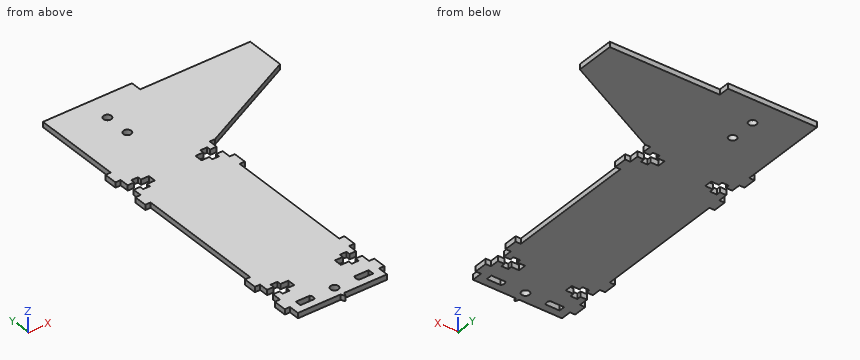
```python
from build123d import *

# Parameters (mm, degrees)
SKETCH_1_R      = 1.5
EXTRUDE_1_DEPTH = 2


with BuildPart() as part:
    # 草图1 → 凸台-拉伸1 (new body)
    with BuildSketch(Plane.XY):
        Polygon((16.993865071, 15.9), (16.993865071, 20), (-16.993865071, 20), (-16.993865071, 15.9), (-16.993865071, -14), (-18.993865071, -14), (-18.993865071, -19), (-16.993865071, -19), (-16.993865071, -22.5), (-14.493865071, -22.5), (-14.493865071, -21), (-11.893865071, -21), (-11.893865071, -22.5), (-8.893865071, -22.5), (-8.893865071, -25.5), (-11.893865071, -25.5), (-11.893865071, -27), (-14.493865071, -27), (-14.493865071, -25.5), (-16.993865071, -25.5), (-16.993865071, -29), (-18.993865071, -29), (-18.993865071, -34), (-16.993865071, -34), (-16.993865071, -84), (-18.993865071, -84), (-18.993865071, -89), (-16.993865071, -89), (-16.993865071, -92.5), (-14.493865071, -92.5), (-14.493865071, -91), (-11.893865071, -91), (-11.893865071, -92.5), (-8.893865071, -92.5), (-8.893865071, -95.5), (-11.893865071, -95.5), (-11.893865071, -97), (-14.493865071, -97), (-14.493865071, -95.5), (-16.993865071, -95.5), (-16.993865071, -99), (-18.993865071, -99), (-18.993865071, -104), (-16.993865071, -104), (-16.993865071, -108), (-0.721190694, -108), (0, -109.5), (0.721190694, -108), (16.993865071, -108), (16.993865071, -104), (18.993865071, -104), (18.993865071, -99), (16.993865071, -99), (16.993865071, -95.5), (14.493865071, -95.5), (14.493865071, -97), (11.893865071, -97), (11.893865071, -95.5), (8.893865071, -95.5), (8.893865071, -92.5), (11.893865071, -92.5), (11.893865071, -91), (14.493865071, -91), (14.493865071, -92.5), (16.993865071, -92.5), (16.993865071, -89), (18.993865071, -89), (18.993865071, -84), (16.993865071, -84), (16.993865071, -34), (18.993865071, -34), (18.993865071, -29), (16.993865071, -29), (16.993865071, -25.5), (14.493865071, -25.5), (14.493865071, -27), (11.893865071, -27), (11.893865071, -25.5), (8.893865071, -25.5), (8.893865071, -22.5), (11.893865071, -22.5), (11.893865071, -21), (14.493865071, -21), (14.493865071, -22.5), (16.993865071, -22.5), (16.993865071, -19), (18.993865071, -19), (58.993865071, 0.9), (58.993865071, 15.9), align=None)
        with Locations((0, -104)):
            Circle(SKETCH_1_R, mode=Mode.SUBTRACT)
        Circle(SKETCH_1_R, mode=Mode.SUBTRACT)
        with Locations((0, 10)):
            Circle(SKETCH_1_R, mode=Mode.SUBTRACT)
        with BuildLine():
            Line((-13.9, -102.85), (-8.6, -102.85))
            ThreePointArc((-8.6, -102.85), (-8.123654403, -104), (-8.6, -105.15))
            Line((-8.6, -105.15), (-13.9, -105.15))
            Line((-13.9, -105.15), (-13.9, -102.85))
        make_face(mode=Mode.SUBTRACT)
        with BuildLine():
            Line((13.9, -105.15), (8.6, -105.15))
            ThreePointArc((8.6, -105.15), (8.123654403, -104), (8.6, -102.85))
            Line((8.6, -102.85), (13.9, -102.85))
            Line((13.9, -102.85), (13.9, -105.15))
        make_face(mode=Mode.SUBTRACT)
    extrude(amount=EXTRUDE_1_DEPTH)


solid = part.part
```
Design review of the part built by this model. Coordinates are the model's own, in mm. Give positions to 0.01 mm unless a question says otherwise; leave off trailing zeros. Loops run counter-clockwise (first coordinate to the right, second up) from the corner with the lowest first, then second, coordinate; pieces in that order, holes last. Notation, with made-up numbers: M 38.5,1 L 84.5,1 A21 ccw 84.5,8 Z; hole C -24,-23.5 d5. An arc over 180 degrees is marked long. Return JSON: item names as keys, results as strings. Group by question number.
Item 1: We need section A-A (y = 10). Give the boundary of the cut face in (x, z), and give its area (3 significant figures).
Item 2: We need section C-C (z = 1.6). Give the number of separate pieces and of enclosed holes in the cut face, and give its area (3 significant figures).
Item 3: For probe 1 along Y at (x, z) = (18.5, 1.9); probe 2 along Y at (x, z) = (9, 1.4); probe 3 along X at (y, z) = (-96, 0.35), list the stretches that pass through material, from the lowest coordinate up.
Item 4: Insertion check: pin 1 Ø0.6 at (x, z) = (-16, 1) entering from -Y; pin 2 Ø0.6 at (y, z) = (-32, 0.5) entering from +X; pin 3 Ø1 at (y, z) = (-28, 0.5) entering from +X. Each pin has a flat end and moves straight along its axis. Give the tip position at first contact, or say it passes through.
Item 5: We need section B-B (y = -50). Give the boundary of the cut face in (x, z), and give its area (3 significant figures).
Item 6: We need section D-D (x = 46). Give the boundary of the cut face in (y, z).
Output:
{
 "1": {"outline": "M -16.99,0 L -1.5,0 L -1.5,2 L -16.99,2 Z; M 1.5,0 L 58.99,0 L 58.99,2 L 1.5,2 Z", "area": "146 mm^2"},
 "2": {"separate pieces": "1", "enclosed holes": "5", "area": "5,310 mm^2"},
 "3": {"probe 1": "y = -104 to -99, -89 to -84, -34 to -29, -19 to 15.9", "probe 2": "y = -108 to -105.15, -102.85 to -95.5, -92.5 to -25.5, -22.5 to 20", "probe 3": "x = -16.99 to -14.49, -11.89 to 11.89, 14.49 to 16.99"},
 "4": {"pin 1": "stops at y = -108", "pin 2": "stops at x = 18.99", "pin 3": "stops at x = 16.99"},
 "5": {"outline": "M -16.99,0 L 16.99,0 L 16.99,2 L -16.99,2 Z", "area": "68.0 mm^2"},
 "6": {"outline": "M -5.56,0 L 15.9,0 L 15.9,2 L -5.56,2 Z"}
}
